Geometry: final body of the model. Coordinates: model frame, mm. Face numbers are marked on the shaded views. A direction names the side the tool comes from. Give positions to 0.01 mm unless a question says otherwise; leave off trailing zeros. Write each loop counter-clockwise with the first axis right and the second up, starting at its lowest first coordinate (ties: lowest second). Pieces come first, ordered by that corner, then holes. Notation, with made-up numbers: M 58.5,-28.5 L 71.5,-28.5 A19 cw 71.5,-11.5 Z; hole C 65.25,-18.5 d3. An arc over 180 degrees is marked long. Use a Markdown table: item, result. Add a question column.
(1) Cut plane B-B (y = -26). Output: boundary loops of the cut face in (x, z).
(2) Cut plane A-A (y = 5). Output: boundary loops of the cut face in (x, z), plus the area to 3 significant figures.
(3) Material intervals for L1, parallel to Y at x = -0.25, z = -4.75; L2, parallel to X at y = -6.5, z = 0.25; L3, parallel to X at y = -26.5, z = -2.25, sorted ascending.
(4) Draft query along Z for the marked faces 1, 2 and 3. Return one class per face: released by +Z, released by -Z, zero draft, split by the parting line, or undercut.
(5) Pin query (flat end, axial travel): pin 1 Ø1.5 at (x, z) = (3, 4.5) entering from -Y; pin 2 Ø1.2 at (x, z) = (-1, -2) entering from +Y; pin 3 Ø2 at (y, z) = (-12.5, 3) entering from -X. Return the tip coordinate at first contact, or that it passes through.
(6) Reachability of the marked faces 4, 5 and 6 from +Z, -Z, +X, -X, +Y, -Y: full face, straight path, thin tool, end or side. Return the list, or none.
```python
from build123d import *

# Parameters (mm, degrees)
ESQUISSE2_R             = 4
BASE_EXTRUSION_DEPTH    = 45
CHANFREIN1_SIZE         = 0.8
ENL_V_MAT_EXTRU_1_DEPTH = 4


with BuildPart() as part:
    # Esquisse2 → Base-Extrusion (new body)
    with BuildSketch(Plane(origin=(0, 0, 0), x_dir=(1, 0, 0), z_dir=(0, 1, 0))):
        with Locations(Location((0, 0, 0), (0, 0, 270))):  # turned: the seam where the file's is
            Circle(ESQUISSE2_R)
    extrude(amount=-BASE_EXTRUSION_DEPTH)

    # Chanfrein1
    chanfrein1_edges = [part.edges().sort_by_distance(p)[0] for p in [
        (0, -45, -4),
    ]]
    chamfer(chanfrein1_edges, length=CHANFREIN1_SIZE)

    # Esquisse5 → Boss.-Révol.1 (revolve)
    with BuildSketch(Plane.XY, mode=Mode.PRIVATE) as boss_r_vol_1_sk:
        with BuildLine():
            Line((3, 8), (3, 4))
            Line((3, 4), (0, 2.267949192))
            Line((0, 2.267949192), (0, 0))
            Line((0, 0), (6.5, 0))
            Line((6.5, 0), (6.5, 7.2))
            ThreePointArc((6.5, 7.2), (6.265685425, 7.765685425), (5.7, 8))
            Line((5.7, 8), (3, 8))
        make_face()
    revolve(boss_r_vol_1_sk.sketch.rotate(Axis((0, 8, 0), (0, -1, 0)), 90), axis=Axis((0, 8, 0), (0, -1, 0)))  # turned: the seam where the file's is

    # Esquisse7 → Enlèv. mat.-Extru.1 (cut)
    with BuildSketch(Plane(origin=(0, 8, 0), x_dir=(-1, 0, 0), z_dir=(0, 1, 0))):
        Polygon((1.732050808, 3), (-1.732050808, 3), (-3.464101615, 0), (-1.732050808, -3), (1.732050808, -3), (3.464101615, 0), align=None)
    extrude(amount=-ENL_V_MAT_EXTRU_1_DEPTH, mode=Mode.SUBTRACT)


solid = part.part
```
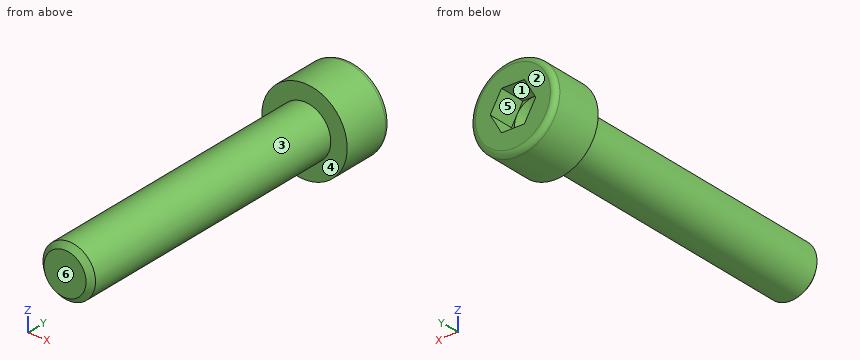
Answer list:
| question | item | result |
|---|---|---|
| 1 | outline | C 0,0 d8 |
| 2 | outline | C 0,0 d13; hole M -3.46,0 L -1.73,-3 L 1.73,-3 L 3.46,0 L 1.73,3 L -1.73,3 Z |
| 2 | area | 102 mm² |
| 3 | L1 | 0 to 8 |
| 3 | L2 | -3.99 to 3.99 |
| 3 | L3 | -3.31 to 3.31 |
| 4 | face 1 | undercut |
| 4 | face 2 | zero draft |
| 4 | face 3 | split by the parting line |
| 5 | pin 1 | y = 0 |
| 5 | pin 2 | y = 3.91 |
| 5 | pin 3 | x = -3.46 |
| 6 | face 4 | -Y |
| 6 | face 5 | +Y |
| 6 | face 6 | +Z, -Z, +X, -X, -Y |
